Source: CAD feature listing. Evaluate the final solid. Frame: model axes, mm. Face numbers are marked on the shaded views. A direction names the side the tool comes from. Coordinates: 2 decimals unless noted, no trailing zeros. Loops run counter-clockwise (first coordinate to the right, second up) from the corner with the lowest first, then second, coordinate; pieces in that order, holes last.
Item 1: Section query A-A, the plane z = 0. Return the cut outline in (x, y).
Item 2: Section query C-C, the plane y = -5.7. Return the cut outline in (x, z).
Item 3: Pin query (flat end, axial travel): pin 1 Ø1.9 at (x, y) = (-4.8, -5.7) entering from -Z; pin 2 Ø1.2 at (y, z) = (-3, 2) entering from +X; pin 3 Ø0.6 at (y, z) = (-4.5, 2.5) entering from -X; pin 4 Ø1.6 at (x, z) = (-1.5, 8) entering from -Y. Return the tip coordinate at first contact, or that it passes through.
Item 4: Reachability of the marked faces 1, 2, 3 and 4 from +Z, -Z, +X, -X, +Y, -Y: full face, straight path, thin tool, end or side. Return the list, or none.
Item 5: Line query: probe 1 along Z at (x, y) = (-2, -8.25); probe 2 along X at (y, z) = (7, 0); probe 3 along X at (y, z) = (11.15, 0). Output: solid intervals per line, ascending.
Item 6: Section query D-D, the plane y = 9.5. Return the cut outline in (x, z), then the cut area to 3 significant figures.
Item 7: Pull-direction query (X, two-part tool) for the marked faces 5, 6 and 7; classes: +X half, -X half, draft (parallel to the pull), parting line (faces both ways), or undercut.
```python
from build123d import *
from build123d.topology import SkipClean

# Parameters (mm, degrees)
SKETCH_9_R          = 9
EXTRUDE_4_DEPTH     = 3
SKETCH_10_R         = 7
EXTRUDE_5_DEPTH     = 6
SKETCH_11_W         = 16
SKETCH_11_H         = 3
EXTRUDE_6_DEPTH     = 10
SKETCH_12_R         = 1.6
CUT_EXTRUDE_3_DEPTH = 20.059118553
SKETCH_13_R         = 12.035495365
SKETCH_13_R_2       = 9
CUT_EXTRUDE_4_DEPTH = 30
FILLET_1_R          = 3
SKETCH_14_R         = 1.15
CUT_EXTRUDE_5_DEPTH = 30
SKETCH_15_W         = 22.433214128
SKETCH_15_H         = 3.5
CUT_EXTRUDE_6_DEPTH = 20
SKETCH_17_R         = 12.049205959
SKETCH_17_R_2       = 8.5
CUT_EXTRUDE_7_DEPTH = 20
SKETCH_18_R         = 9.534410067
SKETCH_18_R_2       = 5.9
CUT_EXTRUDE_8_DEPTH = 2.2
SKETCH_20_W         = 6
SKETCH_20_H         = 6
SKETCH_20_R         = 1.15
EXTRUDE_7_DEPTH     = 6
CHAMFER_1_SIZE      = 2


with BuildPart() as part:
    # Эскиз9 → Бобышка-Вытянуть4 (new body)
    with BuildSketch(Plane(origin=(0, 0, 0), x_dir=(1, 0, 0), z_dir=(0, 1, 0))):
        with Locations(Location((0, 0, 0), (0, 0, 270))):
            Circle(SKETCH_9_R)
    extrude(amount=EXTRUDE_4_DEPTH)

    # Эскиз10 → Бобышка-Вытянуть5 (add)
    with BuildSketch(Plane(origin=(0, 3, 0), x_dir=(1, 0, 0), z_dir=(0, 1, 0))):
        with Locations(Location((0, 0, 0), (0, 0, 270))):
            Circle(SKETCH_10_R)
    extrude(amount=EXTRUDE_5_DEPTH)

    # Эскиз11 → Бобышка-Вытянуть6 (add)
    with BuildSketch(Plane.XZ):
        with Locations((0, -3)):
            Rectangle(SKETCH_11_W, SKETCH_11_H)
        with Locations((0, 3)):
            Rectangle(SKETCH_11_W, SKETCH_11_H)
    extrude(amount=EXTRUDE_6_DEPTH)

    # Эскиз12 → Вырез-Вытянуть3 (cut, through all)
    with BuildSketch(Plane.XY.offset(4.5)):
        with Locations((-4.8, -5.7)):
            Circle(SKETCH_12_R)
        with Locations((4.8, -5.7)):
            Circle(SKETCH_12_R)
    extrude(amount=-CUT_EXTRUDE_3_DEPTH, mode=Mode.SUBTRACT)

    # Эскиз13 → Вырез-Вытянуть4 (cut)
    with SkipClean():  # the faces are left unmerged after this step: merging them gives an invalid solid
        with BuildSketch(Plane.XZ.offset(10)):
            Circle(SKETCH_13_R)
            with Locations(Location((0, 0, 0), (0, 0, 210))):
                Circle(SKETCH_13_R_2, mode=Mode.SUBTRACT)
        extrude(amount=-CUT_EXTRUDE_4_DEPTH, mode=Mode.SUBTRACT)
    add(part.part.scale(1), mode=Mode.REPLACE)  # the faces are merged on a copy

    # Скругление1
    fillet_1_edges = [part.edges().sort_by_distance(p)[0] for p in [
        (-8, -10, -2.811552813),
        (8, -10, -2.811552813),
        (8, -10, 2.811552813),
        (-8, -10, 2.811552813),
    ]]
    fillet(fillet_1_edges, radius=FILLET_1_R)

    # Эскиз14 → Вырез-Вытянуть5 (cut)
    with BuildSketch(Plane.XZ):
        with Locations(Location((0, 0, 0), (0, 0, 270))):
            Circle(SKETCH_14_R)
    extrude(amount=-CUT_EXTRUDE_5_DEPTH, mode=Mode.SUBTRACT)

    # Эскиз15 → Вырез-Вытянуть6 (cut)
    with BuildSketch(Plane.XZ):
        Rectangle(SKETCH_15_W, SKETCH_15_H)
    extrude(amount=CUT_EXTRUDE_6_DEPTH, mode=Mode.SUBTRACT)

    # Эскиз17 → Вырез-Вытянуть7 (cut)
    with BuildSketch(Plane.XZ.offset(10)):
        Circle(SKETCH_17_R)
        with Locations(Location((0, 0, 0), (0, 0, 328.034281249))):
            Circle(SKETCH_17_R_2, mode=Mode.SUBTRACT)
    extrude(amount=-CUT_EXTRUDE_7_DEPTH, mode=Mode.SUBTRACT)

    # Эскиз18 → Вырез-Вытянуть8 (cut)
    with BuildSketch(Plane(origin=(0, 9, 0), x_dir=(1, 0, 0), z_dir=(0, 1, 0))):
        Circle(SKETCH_18_R)
        with Locations(Location((0, 0, 0), (0, 0, 270))):
            Circle(SKETCH_18_R_2, mode=Mode.SUBTRACT)
    extrude(amount=-CUT_EXTRUDE_8_DEPTH, mode=Mode.SUBTRACT)

    # Эскиз20 → Бобышка-Вытянуть7 (add)
    with SkipClean():  # the faces are left unmerged after this step: merging them gives an invalid solid
        with BuildSketch(Plane(origin=(0, 9, 0), x_dir=(1, 0, 0), z_dir=(0, 1, 0))):
            Rectangle(SKETCH_20_W, SKETCH_20_H)
            with Locations(Location((0, 0, 0), (0, 0, 90))):
                Circle(SKETCH_20_R, mode=Mode.SUBTRACT)
        extrude(amount=EXTRUDE_7_DEPTH)

    # Фаска1
    # the kernel refuses this chamfer: 2 mm, written as the material it adds along each edge
    with BuildSketch(Plane(origin=(12.354468527, 0, -4.5), x_dir=(0, -0.9996219169112968, 0.027495876610586494), z_dir=(-1, 0, 0))) as chamfer_1_piece_1_section:
        Polygon((CHAMFER_1_SIZE * 0.999621916911, -CHAMFER_1_SIZE * 0.0274958766106), (-CHAMFER_1_SIZE * 0.0274958766106, -CHAMFER_1_SIZE * 0.999621916911), (0, 0), align=None)
    chamfer_1_piece_1 = extrude(amount=24.708937054, mode=Mode.PRIVATE)
    chamfer_1_piece_1 = chamfer_1_piece_1 & Plane(origin=(0, -0.675834344, 0), x_dir=(0.8483650059896506, 0, -0.5294117647088891), z_dir=(0, -1, 0)) * Cylinder(8.5, 58, mode=Mode.PRIVATE)
    add(chamfer_1_piece_1)
    with BuildSketch(Plane(origin=(-12.354468527, 0, 4.5), x_dir=(0, -0.9996219169112968, -0.027495876610586494), z_dir=(1, 0, 0))) as chamfer_1_piece_2_section:
        Polygon((CHAMFER_1_SIZE * 0.999621916911, -CHAMFER_1_SIZE * 0.0274958766106), (-CHAMFER_1_SIZE * 0.0274958766106, -CHAMFER_1_SIZE * 0.999621916911), (0, 0), align=None)
    chamfer_1_piece_2 = extrude(amount=24.708937054, mode=Mode.PRIVATE)
    chamfer_1_piece_2 = chamfer_1_piece_2 & Plane(origin=(0, -0.675834348, 0), x_dir=(0.8483650059896506, 0, -0.5294117647088891), z_dir=(0, -1, 0)) * Cylinder(8.5, 58, mode=Mode.PRIVATE)
    add(chamfer_1_piece_2)


solid = part.part
```
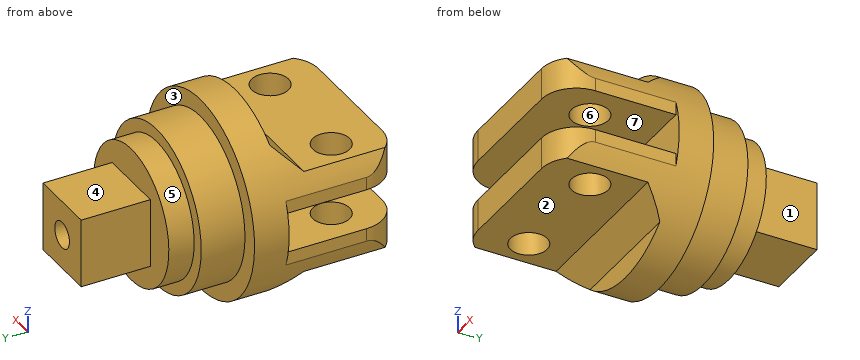
Verdict:
1. outline: (-8.5, 0) - (-1.15, 0) - (-1.15, 15) - (-3, 15) - (-3, 9) - (-5.9, 9) - (-5.9, 6.8) - (-7, 6.8) - (-7, 3) - (-8.5, 3) - close; (1.15, 0) - (8.5, 0) - (8.5, 3) - (7, 3) - (7, 6.8) - (5.9, 6.8) - (5.9, 9) - (3, 9) - (3, 15) - (1.15, 15) - close
2. outline: (-8, -2.87) arc R8.5 ccw to (-7.21, -4.5) - (-6.4, -4.5) - (-6.4, -1.75) - (-8, -1.75) - close; (-8, 1.75) - (-6.4, 1.75) - (-6.4, 4.5) - (-7.21, 4.5) arc R8.5 ccw to (-8, 2.87) - close; (-3.2, -4.5) - (3.2, -4.5) - (3.2, -1.75) - (-3.2, -1.75) - close; (-3.2, 1.75) - (3.2, 1.75) - (3.2, 4.5) - (-3.2, 4.5) - close; (6.4, -4.5) - (7.21, -4.5) arc R8.5 ccw to (8, -2.87) - (8, -1.75) - (6.4, -1.75) - close; (6.4, 1.75) - (8, 1.75) - (8, 2.87) arc R8.5 ccw to (7.21, 4.5) - (6.4, 4.5) - close
3. pin 1: passes through
3. pin 2: stops at x = 8
3. pin 3: stops at x = -8
3. pin 4: stops at y = 0
4. face 1: +Z, -Z, +X, +Y
4. face 2: -Z, +X, -X, -Y
4. face 3: +Y
4. face 4: +Z, +X, -X, +Y
5. probe 1: z = -4.5 to -1.75, 1.75 to 4.5
5. probe 2: x = -5.9 to -1.15, 1.15 to 5.9
5. probe 3: x = -3 to -1.15, 1.15 to 3
6. outline: (-3, -3) - (3, -3) - (3, 3) - (-3, 3) - close; hole circle Ø2.3 at (0, 0)
6. area: 31.8 mm2
7. face 5: parting line
7. face 6: undercut
7. face 7: draft
